from build123d import *

# Parameters (mm, degrees)
SKETCH1_R                = 5
BOSS_EXTRUDE1_DEPTH      = 3.175
SKETCH2_W                = 7.669126603
SKETCH2_H                = 3.535914735
BOSS_EXTRUDE2_DEPTH      = 3.175
F_8_0_8_DIAMETER_HOLE1_D = 8


with BuildPart() as part:
    # Sketch1 → Boss-Extrude1 (new body)
    with BuildSketch(Plane(origin=(0, 0, 0), x_dir=(1, 0, 0), z_dir=(0, 1, 0))):
        Circle(SKETCH1_R)
    extrude(amount=BOSS_EXTRUDE1_DEPTH)

    # Sketch2 → Boss-Extrude2 (add)
    with BuildSketch(Plane(origin=(0, 3.175, 0), x_dir=(1, 0, 0), z_dir=(0, 1, 0))):
        with Locations((-1.383775104, 4.607725038)):
            Rectangle(SKETCH2_W, SKETCH2_H)
    extrude(amount=-BOSS_EXTRUDE2_DEPTH)

    # Ø8.0 (8) Diameter Hole1 (through all)
    with Locations(Plane(origin=(0, 3.175, 0), x_dir=(1, 0, 0), z_dir=(0, 1, 0))):
        with Locations((-0.606472724, 0.48661405)):
            Hole(F_8_0_8_DIAMETER_HOLE1_D / 2)


solid = part.part
Source: CAD feature listing. Evaluate the final solid. Frame: model axes, mm. A direction names the side the tool comes from. Coordinates: 2 decimals unless noted, no trailing zeros. Loops run counter-clockwise (first coordinate to the right, second up) from the corner with the lowest first, then second, coordinate; pieces in that order, holes last. Notation, with made-up numbers: (-9.75, -33) -> (42.25, -33) arc R16 cw to (42.25, -19) -> close; hole circle Ø5 at (39, 38). An arc over 180 degrees is marked (long way). Answer in a Markdown table with one row per item. Add a question column.
Q1. Section A-A on z = -1. Return the cut outline in (x, y) (3 decimals), and give its area (3 significant figures).
Q2. Reachability of faces 1 (the face through (2.451, 2, -5)), 2 (the face through (1, 1.6, 4.9)), 3 (the face through (-5, 2, -2.84)) from +Z, -Z, +X, -X, +Y, -Y: full face, straight path, thin tool, end or side. Return the list, or none.
Q3. Contact query for flat-ended pins moving along their axis: pin 1 Ø6 at (x, z) = (4, -5) entering from +Y (3 decimals); pin 2 Ø1.5 at (x, y) = (3.5, 2.5) entering from -Z; pin 3 Ø1.2 at (x, y) = (-5, 2) entering from +Z. Output: stop coordinate, or through.
Q4. Pull-direction query (X, two-part tool) for faces 4 (the face through (-5.218, 2, -5)), 5 (the face through (0.26, 1.57, 3.42)), 6 (the face through (0, 0, -5)); classes: pulls with the +X half, pulls with the -X half, needs draft (parallel to the pull), parting line crosses it, or undercut.
Q5. Section B-B on x = -0.75. Return the cut outline in (y, z) (3 decimals), and give its area (3 significant figures).
Q6. Ray query, line 1 along Z through (x, y) = (0, 3.05); line 2 along X through (y, z) = (0.85, 0.75); line 3 along X through (y, z) = (2.4, -5.75). Return the intervals inside material, ascending.
Q7. Section C-C on y = 2. Return the cut outline in (x, z).
Computed values:
| question | item | result |
|---|---|---|
| 1 | outline | (-4.899, 0) -> (-4.573, 0) -> (-4.573, 3.175) -> (-4.899, 3.175) -> close; (3.36, 0) -> (4.899, 0) -> (4.899, 3.175) -> (3.36, 3.175) -> close |
| 1 | area | 5.92 mm^2 |
| 2 | face 1 | -Z, +X, +Y, -Y |
| 2 | face 2 | +Y, -Y |
| 2 | face 3 | -X, +Y, -Y |
| 3 | pin 1 | stops at y = 3.175 |
| 3 | pin 2 | stops at z = -4.18 |
| 3 | pin 3 | stops at z = 2.37 |
| 4 | face 4 | pulls with the -X half |
| 4 | face 5 | undercut |
| 4 | face 6 | needs draft |
| 5 | outline | (0, -6.376) -> (3.175, -6.376) -> (3.175, -4.484) -> (0, -4.484) -> close; (0, 3.511) -> (3.175, 3.511) -> (3.175, 4.943) -> (0, 4.943) -> close |
| 5 | area | 10.6 mm^2 |
| 6 | line 1 | z = -6.38 to -4.44, 3.47 to 5 |
| 6 | line 2 | x = -4.94 to -4.41, 3.2 to 4.94 |
| 6 | line 3 | x = -5.22 to 2.45 |
| 7 | outline | (-5.22, -6.38) -> (2.45, -6.38) -> (2.45, -4.36) arc R5 ccw (long way) to (-4.12, -2.84) -> (-5.22, -2.84) -> close; hole circle Ø8 at (-0.61, -0.49) |
